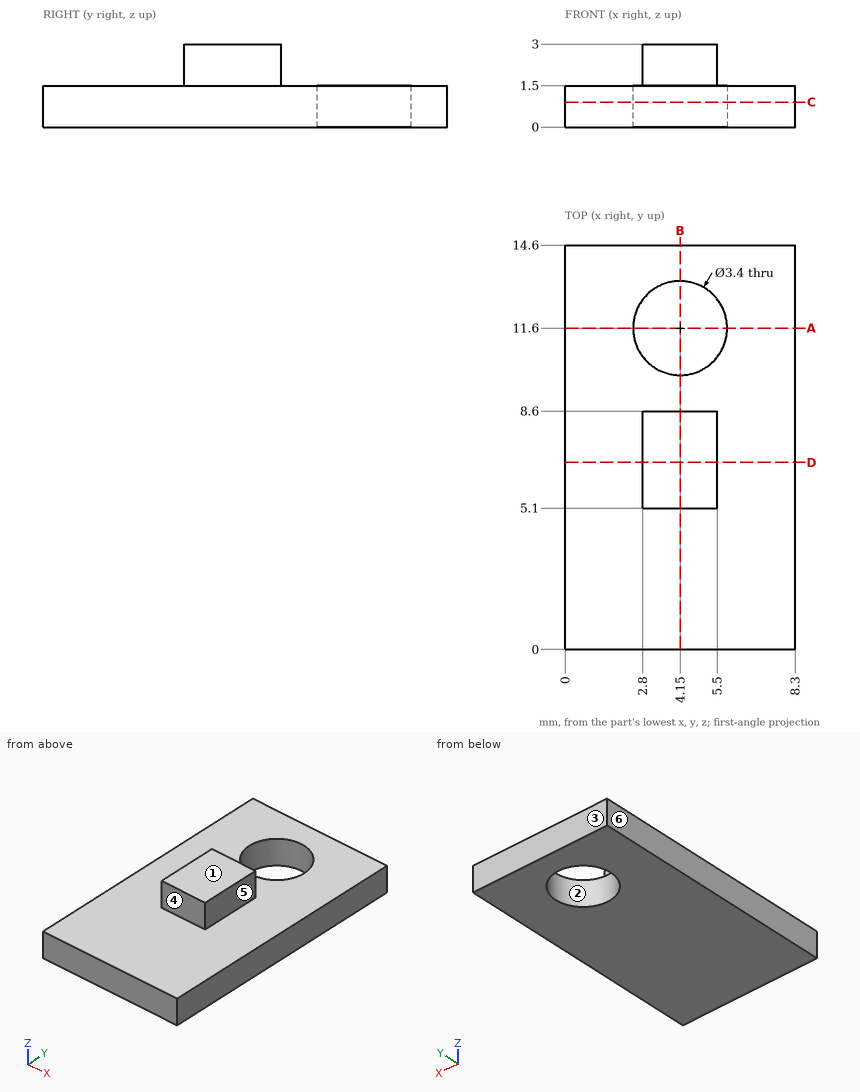
Check sheet for the drawn part. Datum: minimum x, y, z corner. Units: mm. A direction names the side the tool comes from. Coordinates: 2 decimals unless noted, no trailing zeros. Order: outer loops, then holes, each group sorted by start corner. A loop starts at its lowest first (then second) coordinate and runs counter-clockwise, first axis right, second up. Notation, with made-up numbers: M 63,6.5 L 78,6.5 A21 cw 78,32.5 Z; hole C 61,-34 d9. An arc over 180 degrees is marked long. One line per question, with ' | ' between items. Start each with the question number.
Item 1: Cross-section at A-A on y = 11.6. Enter the section's corners in (x, z), then the cut area to 3 significant figures.
Item 2: Draft check along Y on the marked faces 1, 2 and 3. Enter one of: pulls with the +Y half, pulls with the -Y half, needs draft (parallel to the pull), parting line crosses it, or undercut.
Item 3: Gauge pin test, flat ends, axial feed: pin 1 (2 mm diameter, centred on x = 2, y = 2.5, fed in from -Z); pin 2 (0.8 mm diameter, centred on y = 7.5, z = 2, fed in from +X); pin 3 (1.6 mm diameter, centred on x = 4.5, z = 2.5, fed in from -Y); pin 4 (0.8 mm diameter, centred on x = 4, z = 2, fed in from +Y). Record the tip position at first contact, or that the pin passes through.
Item 4: Cross-section at B-B on x = 4.15. Enter the section's corners in (y, z), then the cut area to 4 significant figures.
Item 5: Cross-section at C-C on z = 0.9. Enter the section's corners in (x, y), then the cut area to 3 significant figures.
Item 6: Material ranges on L1, parallel to Y at x = 4.15, z = 0.7; L2, parallel to Y at x = 3, z = 2.35; L3, parallel to Z at x = 1.5, y = 6, recorded low to high. Write a range as [from, to].
Item 7: Cross-section at D-D on y = 6.75. Enter the section's corners in (x, z), then the cut area to 3 significant figures.
Item 8: Set-up check for the marked faces 4, 5 and 6: record each of +Z, -Z, +X, -X, +Y, -Y from which the full face is reachable in a straight line by a thin tool's end or side.
Findings:
1) outline: M 0,0 L 2.45,0 L 2.45,1.5 L 0,1.5 Z; M 5.85,0 L 8.3,0 L 8.3,1.5 L 5.85,1.5 Z | area: 7.35 mm²
2) face 1: needs draft | face 2: undercut | face 3: pulls with the +Y half
3) pin 1: stops at z = 0 | pin 2: stops at x = 5.5 | pin 3: stops at y = 5.1 | pin 4: stops at y = 8.6
4) outline: M 0,0 L 9.9,0 L 9.9,1.5 L 8.6,1.5 L 8.6,3 L 5.1,3 L 5.1,1.5 L 0,1.5 Z; M 13.3,0 L 14.6,0 L 14.6,1.5 L 13.3,1.5 Z | area: 22.05 mm²
5) outline: M 0,0 L 8.3,0 L 8.3,14.6 L 0,14.6 Z; hole C 4.15,11.6 d3.4 | area: 112 mm²
6) L1: y = [0, 9.9], [13.3, 14.6] | L2: y = [5.1, 8.6] | L3: z = [0, 1.5]
7) outline: M 0,0 L 8.3,0 L 8.3,1.5 L 5.5,1.5 L 5.5,3 L 2.8,3 L 2.8,1.5 L 0,1.5 Z | area: 16.5 mm²
8) face 4: +Z, +X, -X, -Y | face 5: +Z, +X, +Y, -Y | face 6: +Z, -Z, -X, +Y, -Y
